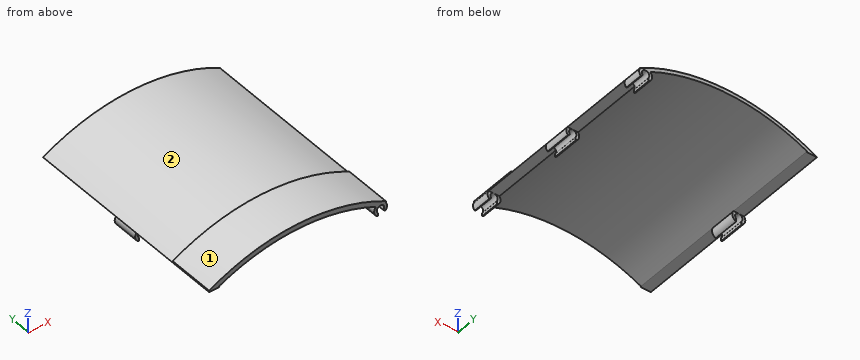
from build123d import *

# Parameters (mm, degrees)
EXTRUDE_1_DEPTH     = 114
EXTRUDE_2_DEPTH     = 25
SKETCH_4_W          = 16.237843285
SKETCH_4_H          = 40
SKETCH_4_W_2        = 18.842025699
SKETCH_4_H_2        = 50
SKETCH_4_W_3        = 19.914336105
CUT_EXTRUDE_1_DEPTH = 20


with BuildPart() as part:
    # 草图1 → 凸台-拉伸1 (new body)
    with BuildSketch(Plane(origin=(0, 0, 0), x_dir=(1, 0, 0), z_dir=(0, 1, 0))):
        with BuildLine():
            Line((90.5, 3.322875656), (90.5, 5.16227766))
            ThreePointArc((90.5, 5.16227766), (88.549473904, 2.586404006), (89.539550125, -0.489214015))
            ThreePointArc((89.539550125, -0.489214015), (47, -10.203390265), (4.460449875, -0.489214015))
            ThreePointArc((4.460449875, -0.489214015), (5.450526096, 2.586404006), (3.5, 5.16227766))
            Line((3.5, 5.16227766), (3.5, 3.322875656))
            ThreePointArc((3.5, 3.322875656), (2, 0), (0.5, 3.322875656))
            Line((0.5, 3.322875656), (0.5, 5.16227766))
            ThreePointArc((0.5, 5.16227766), (-1.382526963, 2.89917259), (-0.872281323, 0))
            ThreePointArc((-0.872281323, 0), (47, -12.203390265), (94.872281323, 0))
            ThreePointArc((94.872281323, 0), (95.494266967, 2.200245764), (94.625, 4.315032397))
            Line((94.625, 4.315032397), (93.5, 3.322875656))
            ThreePointArc((93.5, 3.322875656), (92, 0), (90.5, 3.322875656))
        make_face()
    extrude(amount=EXTRUDE_1_DEPTH)

    # 草图3 → 凸台-拉伸2 (add)
    with BuildSketch(Plane.XZ):
        with BuildLine():
            Line((-0.872281323, 0), (-0.872281323, 0.853303863))
            ThreePointArc((-0.872281323, 0.853303863), (47, 12.953390265), (94.872281323, 0.853303863))
            Line((94.872281323, 0.853303863), (94.872281323, 0))
            ThreePointArc((94.872281323, 0), (47, 12.203390265), (-0.872281323, 0))
        make_face()
    extrude(amount=-EXTRUDE_2_DEPTH)

    # 草图4 → 切除-拉伸1 (cut)
    with BuildSketch(Plane.XY):
        with Locations((92.649785841, 84)):
            Rectangle(SKETCH_4_W, SKETCH_4_H)
        with Locations((92.649785841, 30)):
            Rectangle(SKETCH_4_W, SKETCH_4_H)
        with Locations((0.967246157, 89)):
            Rectangle(SKETCH_4_W_2, SKETCH_4_H_2)
        with Locations((1.50340136, 25)):
            Rectangle(SKETCH_4_W_3, SKETCH_4_H_2)
    extrude(amount=-CUT_EXTRUDE_1_DEPTH, mode=Mode.SUBTRACT)


solid = part.part
Geometry: final body of the model. Coordinates: model frame, mm. Face numbers are marked on the shaded views. A direction names the side the tool comes from. Coordinates: 2 decimals unless noted, no trailing zeros. Loops run counter-clockwise (first coordinate to the right, second up) from the corner with the lowest first, then second, coordinate; pieces in that order, holes last. Notation, with made-up numbers: M -31.75,12.5 L -11.75,12.5 A22 ccw -11.75,19.5 Z; hole C 72,57.5 d6. An arc over 180 degrees is marked long. One line per item, written item: value. Start each with the question number.
1) Pin query (flat end, axial travel): P1, Ø3, axis at x = 2.5, y = 14.5, coming from the -Z side; P2, Ø10, axis at y = 25, z = 7.5, coming from the +X side; P3, Ø10, axis at x = 9, y = 56.5, coming from the -Z side; P4, Ø3.5, axis at x = 92, z = -2, coming from the -Y side. Return the tip coordinate at first contact, or that it passes through.
2) Material intervals for L1, parallel to X at y = 56.25, z = -2; L2, parallel to X at y = 110.25, z = -2; L3, parallel to Z at x = 79.5, y = 13, sorted ascending. Write a range as from..to.
3) Reachability of the marked faces 1 and 2 from +Z, -Z, +X, -X, +Y, -Y: full face, straight path, thin tool, end or side. Return the list, or none.
4) Cut plane A-A (z = -2). Count the separate pieces of the cut face and the enclosed holes in it, then the cut area to 3 significant figures.
5) Cut plane C-C (x = 70). Return loops of the section in (y, z).
6) Cut plane B-B (y = 37.5). Return loops of the section in (x, z).
Evaluation:
1. P1: z = 0
1. P2: x = 91.69
1. P3: z = -4.87
1. P4: through
2. L1: -1.5..0, 4..5.5, 88.5..90, 94..95.5
2. L2: 88.5..90, 94..95.5
2. L3: 4.66..7.57
3. face 1: +Z, +Y, -Y
3. face 2: +Z, +Y
4. separate pieces: 8
4. enclosed holes: 0
4. area: 144 mm^2
5. outline: M 0,7.47 L 114,7.47 L 114,9.52 L 25,9.52 L 25,10.29 L 0,10.29 Z
6. outline: M -0.87,0 L 4.87,0 A3.5 ccw 4.46,0.49 A98 cw 89.54,0.49 A3.5 ccw 89.13,0 L 94.87,0 A100 ccw Z
